Geometry check sheet. Reference: the model listing, model coordinates, mm. A direction names the side the tool comes from. Round coordinates to 2 decimals unless told otherwise and drop trailing zeros. Loops run counter-clockwise (first coordinate to the right, second up) from the corner with the lowest first, then second, coordinate; pieces in that order, holes last. Notation, with made-up numbers: M -4.75,77.25 L 41.25,77.25 A19 ccw 41.25,90.25 Z; hole C 34.5,-11.5 d4. An arc over 180 degrees is marked long. Answer in a Markdown table with one row per item. Add a question column.
```python
from build123d import *

# Parameters (mm, degrees)
SKETCH1_W            = 51
SKETCH1_H            = 21.2
BOSS_EXTRUDE1_DEPTH  = 3
SKETCH2_W            = 39
SKETCH2_H            = 9.2
SKETCH2_W_2          = 33
SKETCH2_H_2          = 3.2
BOSS_EXTRUDE2_DEPTH  = 9
M3_CLEARANCE_HOLE1_D = 3.6
M3_CLEARANCE_HOLE2_D = 3.6


with BuildPart() as part:
    # Sketch1 → Boss-Extrude1 (new body)
    with BuildSketch(Plane(origin=(0, 0, 0), x_dir=(1, 0, 0), z_dir=(0, 1, 0))):
        with Locations((25.5, 10.6)):
            Rectangle(SKETCH1_W, SKETCH1_H)
    extrude(amount=BOSS_EXTRUDE1_DEPTH)

    # Sketch2 → Boss-Extrude2 (add)
    with BuildSketch(Plane(origin=(0, 3, 0), x_dir=(1, 0, 0), z_dir=(0, 1, 0))):
        with Locations((25.5, 10.6)):
            Rectangle(SKETCH2_W, SKETCH2_H)
        with Locations((25.5, 10.6)):
            Rectangle(SKETCH2_W_2, SKETCH2_H_2, mode=Mode.SUBTRACT)
    extrude(amount=BOSS_EXTRUDE2_DEPTH)

    # M3 Clearance Hole1 (through all)
    with Locations(Plane(origin=(0, 3, 0), x_dir=(1, 0, 0), z_dir=(0, 1, 0))):
        with Locations((3, 18.2), (48, 18.2), (48, 3), (3, 3)):
            Hole(M3_CLEARANCE_HOLE1_D / 2)

    # M3 Clearance Hole2 (through all)
    with Locations(Plane.XY.offset(-6)):
        with Locations((13, 7.5), (38, 7.5)):
            Hole(M3_CLEARANCE_HOLE2_D / 2)


solid = part.part
```
1) Cross-section at C-C, the plane y = 2. Record the boundary of the cut face in (x, z).
2) Cross-section at A-A, the plane x = 13. Record the boundary of the cut face in (y, z), plus the area to 3 significant figures.
3) Draft check along Y on faces 4 (the flat face through (25, 0, -11)), 5 (the flat face through (25, 1, -21.2)), 6 (the cylindrical face through (37.169, 5.903, -13.721)), 7 (the flat face through (25, 12, -13)). Enter one of: +Y half, -Y half, draft (parallel to the pull), parting line (faces both ways), or undercut.
4) Thickness scan on L1, parallel to Z at x = 48, y = 2.15; L2, parallel to Z at x = 34, y = 5.5; L3, parallel to Y at x = 38, z = -14.5. Record the ranges inside material, lowest first. Write a range as [from, to].
5) Set-up check for faces 1 (the flat face through (25, 7, -15.2)), 2 (the flat face through (9, 7, -11)), 3 (the flat face through (6, 7, -11)): record each of +Z, -Z, +X, -X, +Y, -Y from which the full face is reachable in a straight line by a thin tool's end or side.
6) Cross-section at B-B, the plane z = -18.2. Record the boundary of the cut face in (x, y).
7) Cross-section at D-D, the plane x = 41. Record the boundary of the cut face in (y, z).
8) Go/stop test with flat-tipped pins: pin 1 (4.5 mm diameter, centred on x = 13, y = 7.5, fed in from +Z); pin 2 (7 mm diameter, centred on y = 7, z = -9, fed in from -X); pin 3 (4 mm diameter, centred on x = 3, z = -18.2, fed in from +Y). Record where each tip stops, or that it passes through.
Worked answers:
| question | item | result |
|---|---|---|
| 1 | outline | M 0,-21.2 L 51,-21.2 L 51,0 L 0,0 Z; hole C 3,-18.2 d3.6; hole C 3,-3 d3.6; hole C 48,-18.2 d3.6; hole C 48,-3 d3.6 |
| 2 | outline | M 0,-21.2 L 3,-21.2 L 3,-15.2 L 5.7,-15.2 L 5.7,-12.2 L 3,-12.2 L 3,-9 L 5.7,-9 L 5.7,-6 L 3,-6 L 3,0 L 0,0 Z; M 9.3,-15.2 L 12,-15.2 L 12,-12.2 L 9.3,-12.2 Z; M 9.3,-9 L 12,-9 L 12,-6 L 9.3,-6 Z |
| 2 | area | 96.0 mm2 |
| 3 | face 4 | -Y half |
| 3 | face 5 | draft |
| 3 | face 6 | undercut |
| 3 | face 7 | +Y half |
| 4 | L1 | z = [-21.2, -20], [-16.4, -4.8], [-1.2, 0] |
| 4 | L2 | z = [-15.2, -12.2], [-9, -6] |
| 4 | L3 | y = [0, 5.7], [9.3, 12] |
| 5 | face 1 | -Z, +X, -X, +Y |
| 5 | face 2 | +Y |
| 5 | face 3 | +Z, -Z, -X, +Y |
| 6 | outline | M 0,0 L 1.2,0 L 1.2,3 L 0,3 Z; M 4.8,0 L 46.2,0 L 46.2,3 L 4.8,3 Z; M 49.8,0 L 51,0 L 51,3 L 49.8,3 Z |
| 7 | outline | M 0,-21.2 L 3,-21.2 L 3,-15.2 L 12,-15.2 L 12,-12.2 L 3,-12.2 L 3,-9 L 12,-9 L 12,-6 L 3,-6 L 3,0 L 0,0 Z |
| 8 | pin 1 | stops at z = -6 |
| 8 | pin 2 | stops at x = 6 |
| 8 | pin 3 | stops at y = 3 |
